Autodesk Inventor part; units mm, degrees
ref_plane "YZ Plane" through (0, 0, 0) normal (1, 0, 0) x (0, 1, 0)
ref_plane "XZ Plane" through (0, 0, 0) normal (0, 1, 0) x (-1, 0, 0)
ref_plane "XY Plane" through (0, 0, 0) normal (0, 0, 1) x (1, 0, 0)
sketch "Skizze2" plane through (0, 0, 0) normal (0, 1, 0) x (-1, 0, 0)
  line L0 (75, 150) -> (-75, 150)
  line L1 (-75, 150) -> (-75, -150)
  line L2 (-75, -150) -> (75, -150)
  line L3 (75, -150) -> (75, 150)
  point P0 (0, 0)
  dimension "d4" = 150
  dimension "d5" = 300
  dimension "d6" = 150
  dimension "d7" = 75
extrude "Extrusion2" add sketch "Skizze2" along normal blind 12
sketch "Skizze3" plane through (-75, 0, -150) normal (-1, 0, 0) x (0, 0, 1)
  line L0 (300, 0) -> (0, 0)
  line L1 (0, 0) -> (300, 0)
  line L2 (300, 0) -> (300, 74)
  line L3 (300, 74) -> (0, 74)
  line L4 (0, 74) -> (0, 0)
  point P0 (150, 0)
  dimension "d10" = 300
  dimension "d11" = 74
extrude "Extrusion3" add sketch "Skizze3" along normal blind 12
sketch "Skizze4" plane through (-75, 0, -150) normal (1, 0, 0) x (0, 0, -1)
  line L0 (-300, 12) -> (-300, 74)
  line L1 (-300, 74) -> (0, 74)
  line L2 (0, 74) -> (0, 62)
  line L3 (0, 62) -> (-300, 62)
  line L4 (-300, 62) -> (-300, 74)
  point P0 (-150, 0)
  dimension "d14" = 300
  dimension "d15" = 12
extrude "Extrusion4" add sketch "Skizze4" along normal blind 150
sketch "Skizze5" plane through (75, 0, 150) normal (0, 0, 1) x (1, 0, 0)
  line L0 (0, 0) -> (-162, 0)
  line L1 (0, 62) -> (0, 74)
  line L2 (-162, 0) -> (0, 0)
  line L3 (0, 0) -> (0, 74)
  line L4 (0, 74) -> (-162, 74)
  line L5 (-162, 74) -> (-162, 0)
  point P0 (-75, 0)
extrude "Extrusion5" add sketch "Skizze5" along normal blind 12
sketch "Skizze6" plane through (75, 0, -150) normal (0, 0, -1) x (-1, 0, 0)
  line L0 (0, 0) -> (0, 12)
  line L1 (162, 74) -> (162, 0)
  line L2 (0, 0) -> (162, 0)
  line L3 (162, 0) -> (162, 74)
  line L4 (162, 74) -> (0, 74)
  line L5 (0, 74) -> (0, 0)
  point P0 (75, 0)
  point P1 (162, 0)
extrude "Extrusion6" add sketch "Skizze6" along normal blind 12
sketch "Skizze7" plane through (-87, 74, 162) normal (0, 1, 0) x (1, 0, 0)
  point P0 (87, 162)
hole "Bohrung1" at (0, 74, 0) direction (0, -1, 0) diameter 12 end through all
sketch "Skizze8" plane through (-75, 0, -150) normal (1, 0, 0) x (0, 0, -1)
  line L0 (0, 62) -> (-300, 62)
  line L1 (0, 12) -> (-300, 12)
  line L2 (-156, 62) -> (-144, 62)
  line L3 (-144, 62) -> (-144, 12)
  line L4 (-144, 12) -> (-156, 12)
  line L5 (-156, 12) -> (-156, 62)
  line L6 (0, 62) -> (0, 12)
  point P0 (-150, 0)
  dimension "d29" = 12
  dimension "d30" = 144
extrude "Extrusion7" add sketch "Skizze8" along normal blind 65 contours L3 L1 L5 L0
sketch "Skizze9" plane through (-10, 0, -150) normal (1, 0, 0) x (0, 0, -1)
  point P0 (-150, 0)
fillet "Rundung1" radius 4 2 edges at (-10, 37, 6) (-10, 37, -6)
sketch "Skizze11" plane through (75, 0, 162) normal (1, 0, 0) x (0, 0, -1)
  line L0 (12, 12) -> (312, 12)
  line L1 (156, 12) -> (168, 12)
  line L2 (168, 12) -> (168, 62)
  line L3 (168, 62) -> (156, 62)
  line L4 (156, 62) -> (156, 12)
  line L5 (156, 12) -> (156, 62)
  point P0 (162, 0)
  dimension "d36" = 12
  dimension "d37" = 50
  dimension "d38" = 0
extrude "Extrusion9" add sketch "Skizze11" against normal blind 65
fillet "Rundung2" radius 4 2 edges at (10, 37, 6) (10, 37, -6)
sketch "Skizze12" plane through (75, 0, 162) normal (1, 0, 0) x (0, 0, -1)
  line L0 (324, 74) -> (0, 74)
  line L1 (0, 74) -> (324, 74)
  line L2 (324, 74) -> (324, 0)
  line L3 (324, 0) -> (0, 0)
  line L4 (0, 0) -> (0, 74)
  point P0 (162, 0)
extrude "Extrusion10" [suppressed]
properties part number "Lenkung"
Geometry: final body of the model. Coordinates: model frame, mm. A direction names the side the tool comes from. Give positions to 0.01 mm unless a question says otherwise; leave off trailing zeros. Write each loop counter-clockwise with the first axis right and the second up, starting at its lowest first coordinate (ties: lowest second). Pieces come first, ordered by that corner, then holes. Notation, with made-up numbers: (81, 11.25) -> (131, 11.25) arc R15 ccw to (131, 38.25) -> close; hole circle Ø11 at (-10.75, 22.25). An arc over 180 degrees is marked (long way). Answer in a Markdown table with one row per item.
(1) Section query A-A on y = 52. Return loops of the section in (x, z), then the cut area to 3 significant figures.
Answers below:
| item | result |
|---|---|
| outline | (-87, -162) -> (75, -162) -> (75, -150) -> (-75, -150) -> (-75, -6) -> (-14, -6) arc R4 ccw to (-10, -2) -> (-10, 2) arc R4 ccw to (-14, 6) -> (-75, 6) -> (-75, 150) -> (75, 150) -> (75, 162) -> (-87, 162) -> close; (10, -2) arc R4 ccw to (14, -6) -> (75, -6) -> (75, 6) -> (14, 6) arc R4 ccw to (10, 2) -> close |
| area | 9,030 mm^2 |
(2) Ray query, line 1 along Z through (x, y) = (24.5, 13.5); line 2 along Y through (x, z) = (-51.5, -26); line 3 along Z through (x, y) = (0, 9.75). Return the intervals inside material, ascending. Write a range as [from, to].
Answers below:
| item | result |
|---|---|
| line 1 | [-162, -150], [-6, 6], [150, 162] |
| line 2 | [0, 12], [62, 74] |
| line 3 | [-162, -6], [6, 162] |
(3) Section query B-B on x = 0. Return loops of the section in (y, z), then the cut area to 3 significant figures.
Answers below:
| item | result |
|---|---|
| outline | (0, -162) -> (74, -162) -> (74, -6) -> (62, -6) -> (62, -150) -> (12, -150) -> (12, -6) -> (0, -6) -> close; (0, 6) -> (12, 6) -> (12, 150) -> (62, 150) -> (62, 6) -> (74, 6) -> (74, 162) -> (0, 162) -> close |
| area | 8,690 mm^2 |
(4) Section query C-C on x = -45. Return loops of the section in (y, z), then the cut area to 3 significant figures.
Answers below:
| item | result |
|---|---|
| outline | (0, -162) -> (74, -162) -> (74, 162) -> (0, 162) -> close; hole (12, -150) -> (62, -150) -> (62, -6) -> (12, -6) -> close; hole (12, 6) -> (62, 6) -> (62, 150) -> (12, 150) -> close |
| area | 9,580 mm^2 |
(5) Section query D-D on z = 137.5. Return loops of the section in (x, y), then the cut area to 3 significant figures.
Answers below:
| item | result |
|---|---|
| outline | (-87, 0) -> (75, 0) -> (75, 12) -> (-75, 12) -> (-75, 62) -> (75, 62) -> (75, 74) -> (-87, 74) -> close |
| area | 4,490 mm^2 |
(6) Draft query along Z for faces 3 (the flat face through (-7, 38, 162)), 4 (the flat face through (45, 37, 6)), 5 (the flat face through (75, 28, 2)). Return one class per face: +Z half, -Z half, draft (parallel to the pull), parting line (faces both ways), or undercut.
Answers below:
| item | result |
|---|---|
| face 3 | +Z half |
| face 4 | undercut |
| face 5 | draft |
(7) Set-up query: faces 1 (the flat face through (-5, 38, -162)), 2 (the flat face through (-1, 37, 150)). Return all of +Z, -Z, +X, -X, +Y, -Y with unobstructed straight access to the full face (end or side cutting, diameter ignored); none if empty.
Answers below:
| item | result |
|---|---|
| face 1 | -Z, +X, -X, +Y, -Y |
| face 2 | +X |
(8) Pin query (flat end, axial travel): pin 1 (10 mm diameter, centred on y = 27, z = -110, fed in from +X); pin 2 (7 mm diameter, centred on x = 0, z = 0, fed in from +Y). Return the tip coordinate at first contact, or that it passes through.
Answers below:
| item | result |
|---|---|
| pin 1 | x = -75 |
| pin 2 | through |
